from build123d import *

# Parameters (mm, degrees)
SKETCH1_R           = 3
BOSS_EXTRUDE1_DEPTH = 3
SKETCH2_R           = 3
CUT_EXTRUDE1_DEPTH  = 3


with BuildPart() as part:
    # Sketch1 → Boss-Extrude1 (new body)
    with BuildSketch(Plane.XY):
        with BuildLine():
            Line((175.891719745, 12.468152866), (350, 6.25))
            ThreePointArc((350, 6.25), (356.25, 0), (350, -6.25))
            Line((350, -6.25), (175.891719745, -12.468152866))
            ThreePointArc((175.891719745, -12.468152866), (175.446144131, -12.492035679), (175, -12.5))
            Line((175, -12.5), (65, -12.5))
            ThreePointArc((65, -12.5), (52.5, 0), (65, 12.5))
            Line((65, 12.5), (175, 12.5))
            ThreePointArc((175, 12.5), (175.446144131, 12.492035679), (175.891719745, 12.468152866))
        make_face()
        with Locations((65, 0)):
            Circle(SKETCH1_R, mode=Mode.SUBTRACT)
        with Locations((80, 0)):
            Circle(SKETCH1_R, mode=Mode.SUBTRACT)
        with Locations((95, 0)):
            Circle(SKETCH1_R, mode=Mode.SUBTRACT)
        with Locations((110, 0)):
            Circle(SKETCH1_R, mode=Mode.SUBTRACT)
        with Locations((125, 0)):
            Circle(SKETCH1_R, mode=Mode.SUBTRACT)
        with Locations((140, 0)):
            Circle(SKETCH1_R, mode=Mode.SUBTRACT)
        with Locations((155, 0)):
            Circle(SKETCH1_R, mode=Mode.SUBTRACT)
        with Locations((170, 0)):
            Circle(SKETCH1_R, mode=Mode.SUBTRACT)
        with Locations((185, 0)):
            Circle(SKETCH1_R, mode=Mode.SUBTRACT)
    extrude(amount=BOSS_EXTRUDE1_DEPTH)

    # Sketch2 → Cut-Extrude1 (cut)
    with BuildSketch(Plane.XY.offset(3)):
        with Locations((200, 0)):
            Circle(SKETCH2_R)
    extrude(amount=-CUT_EXTRUDE1_DEPTH, mode=Mode.SUBTRACT)


solid = part.part
Part model, mm, in its own coordinate system. Give positions to 0.01 mm unless a question says otherwise; leave off trailing zeros. Order: outer loops, then holes, each group sorted by start corner. A loop starts at its lowest first (then second) coordinate and runs counter-clockwise, first axis right, second up. Notation, with made-up numbers: (52, 6.5) -> (105, 6.5) arc R25 cw to (105, 38.5) -> close; hole circle Ø1 at (88, 13.5). An arc over 180 degrees is marked (long way). Use one line per item in the form item = value.
(1) Saw through at D-D (x = 317.5). Write the cut outline in (y, z).
Solution:
outline = (-7.41, 0) -> (7.41, 0) -> (7.41, 3) -> (-7.41, 3) -> close
(2) Saw through at B-B (z = 1.7). Count the separate pieces of the cut face and the enclosed holes in it, then the cut area to 3 significant figures.
Solution:
separate_pieces = 1
enclosed_holes = 10
area = 6,060 mm²
(3) Saw through at A-A (x = 170). Write the cut outline in (y, z).
Solution:
outline = (-12.5, 0) -> (-3, 0) -> (-3, 3) -> (-12.5, 3) -> close; (3, 0) -> (12.5, 0) -> (12.5, 3) -> (3, 3) -> close
(4) Drill centre lines: line 1 (Y direction, x = 155, z = 1.1); line 2 (Y direction, x = 200, z = 2.3); line 3 (X direction, y = -5.5, z = 2). Where is each one in solid material? Low to high. Write a range as from..to.
Solution:
line_1 = -12.5..-3, 3..12.5
line_2 = -11.61..-3, 3..11.61
line_3 = 53.78..352.97
(5) Pull direction X, two halves, no side cores. Call faces 1 (the face through (52.503, -0.275, 1.479)), 2 (the face through (92, 0, 1)), 3 (the face through (207, 0, 3)), 4 (the face through (356.25, 0.14, 1.48)): +X half, -X half, draft (parallel to the pull), parting line (faces both ways), or undercut.
Solution:
face_1 = -X half
face_2 = undercut
face_3 = draft
face_4 = +X half
